Could you check a few things on this model? Use its own coordinates, in mm. A direction names the side the tool comes from. Coordinates: 2 decimals unless noted, no trailing zeros. Loops run counter-clockwise (first coordinate to the right, second up) from the corner with the lowest first, then second, coordinate; pieces in that order, holes last.
1) For faces 1 (the face through (59, 7, -28)), 2 (the face through (48, 6, -17)), 3 (the face through (-54.056, 3.451, 36.542)), which set-ups out of +Z, -Z, +X, -X, +Y, -Y let a thin tool reach every point of the face, with its end or its side?
2) Imagine slicing it at B-B on z = 0. Please give me the cut outline in (x, y).
3) Imagine slicing it at A-A on x = 0. Give the number of separate pieces and of enclosed holes in the cut face, plus the area to 3 significant figures.
4) Imagine slicing it at D-D on z = 67. Please give me the cut outline in (x, y), plus the area to 3 significant figures.
5) Thinking about a two-plate mould opening in Z: for faces 4 (the face through (-59, 7, 28)), 5 (the face through (52, 12, -23)), which applies, released by +Z, released by -Z, zero draft, split by the parting line, or undercut?
6) Imagine slicing it at C-C on y = 2.25. Please give me the cut outline in (x, z), plus the area to 3 significant figures.
7) Will these pins go through, and if not, where does the flat tip stop? P1, Ø7.5, axis at x = -61, z = -35.5, coming from the +Y side; P2, Ø2, axis at y = 9.5, z = 59, coming from the -X side; P3, Ø3, axis at x = 24, y = 4, coming from the +Z side; P4, Ø13, axis at x = -58.02, z = 33.5, coming from the -Y side.
8) If I drill on line 1 along X through (y, z) = (3.1, 0); line 2 along Z through (x, y) = (-61.5, 10.75); line 3 along Z through (x, y) = (3.5, 2), over which ranges is the centre line in solid material (lowest first)?
```python
from build123d import *

# Parameters (mm, degrees)
SKETCH_1_R                    = 77.5
EXTRUDE_D155_DEPTH            = 12
SKETCH_3_R                    = 58
CUT_EXTRUDE_D116_2_DEPTH      = 6
HOLE_WIZARD_M10_6_D           = 10
HOLE_WIZARD_M10_6_CBORE_D     = 15
HOLE_WIZARD_M10_6_CBORE_DEPTH = 5
PATTERN_CIRCULAR_M10_6_COUNT  = 6


with BuildPart() as part:
    # 草图1 → D155 观察窗外盖 (new body)
    with BuildSketch(Plane(origin=(0, 0, 0), x_dir=(1, 0, 0), z_dir=(0, 1, 0))):
        with Locations(Location((0, 0, 0), (0, 0, 270))):
            Circle(SKETCH_1_R)
    extrude(amount=EXTRUDE_D155_DEPTH)

    # 草图2 → D100 内径切除 (revolve, cut)
    with BuildSketch(Plane.XY, mode=Mode.PRIVATE) as cut_revolve_d100_sk:
        Polygon((50, 10), (55, 12), (50, 12), (0, 12), (0, 0), (50, 0), align=None)
    revolve(cut_revolve_d100_sk.sketch.rotate(Axis((0, 0, 0), (0, 1, 0)), 90), axis=Axis((0, 0, 0), (0, 1, 0)), mode=Mode.SUBTRACT)

    # 草图3 → D116*2 橡胶垫(外径) (cut)
    with BuildSketch(Plane.XZ):
        with Locations(Location((0, 0, 0), (0, 0, 270))):
            Circle(SKETCH_3_R)
    extrude(amount=-CUT_EXTRUDE_D116_2_DEPTH, mode=Mode.SUBTRACT)

    # M10*6 柱形沉头孔 (through all)
    with Locations(Plane(origin=(0, 12, 0), x_dir=(1, 0, 0), z_dir=(0, 1, 0))):
        with Locations((0, 67)):
            hole_wizard_m10_6 = CounterBoreHole(HOLE_WIZARD_M10_6_D / 2, HOLE_WIZARD_M10_6_CBORE_D / 2, HOLE_WIZARD_M10_6_CBORE_DEPTH)

    # M10*6 圆周阵列: M10*6 柱形沉头孔 ×6 about axis
    pattern_circular_m10_6_axis = Axis((0, 0, 0), (0, 1, 0))
    for i in range(1, PATTERN_CIRCULAR_M10_6_COUNT):
        add(hole_wizard_m10_6.rotate(pattern_circular_m10_6_axis, i * 360 / PATTERN_CIRCULAR_M10_6_COUNT), mode=Mode.SUBTRACT)


solid = part.part
```
Filled in:
1. face 1: +Y
1. face 2: -Y
1. face 3: +Y, -Y
2. outline: (-77.5, 0) - (-58, 0) - (-58, 6) - (-50, 6) - (-50, 10) - (-55, 12) - (-77.5, 12) - close; (50, 6) - (58, 6) - (58, 0) - (77.5, 0) - (77.5, 12) - (55, 12) - (50, 10) - close
3. separate pieces: 4
3. enclosed holes: 0
3. area: 264 mm2
4. outline: (-38.95, 0) - (-5, 0) - (-5, 7) - (-7.5, 7) - (-7.5, 12) - (-38.95, 12) - close; (5, 0) - (38.95, 0) - (38.95, 12) - (7.5, 12) - (7.5, 7) - (5, 7) - close
4. area: 790 mm2
5. face 4: undercut
5. face 5: zero draft
6. outline: circle Ø155 at (0, 0); hole circle Ø10 at (-58.02, -33.5); hole circle Ø10 at (-58.02, 33.5); hole circle Ø116 at (0, 0); hole circle Ø10 at (0, -67); hole circle Ø10 at (0, 67); hole circle Ø10 at (58.02, -33.5); hole circle Ø10 at (58.02, 33.5)
6. area: 7,830 mm2
7. P1: stops at y = 7
7. P2: stops at x = -51.4
7. P3: stops at z = 74.16
7. P4: stops at y = 0
8. line 1: x = -77.5 to -58, 58 to 77.5
8. line 2: z = -47.16 to -40.15, -26.85 to 26.85, 40.15 to 47.16
8. line 3: z = -77.42 to -70.57, -63.43 to -57.89, 57.89 to 63.43, 70.57 to 77.42
